Can you work these out from the model? Positions are in its coordinate system, mm. Coordinates: 2 decimals unless noted, no trailing zeros. Order: outer loops, then holes, each group sorted by start corner. A loop starts at its lowest first (then second) coordinate and runs counter-clockwise, first axis right, second up. Notation, with made-up numbers: (-16, 64) - (22, 64) arc R29 cw to (22, 94) - close; hole circle Ø9 at (-2.5, 34.25). An arc over 180 degrees is marked (long way). Use a Markdown table: item, result. Add a question column.
(1) I want a section at D-D (x = 29). List the corners of the cut face in (y, z) for me (3 decimals).
(2) If I drill on L1, parallel to Z at x = 19.05, y = 1; L2, parallel to X at y = 1.4, z = 12.7; L3, parallel to X at y = 0.75, z = 89, over which ranges is the centre line in solid material (lowest first)? Write a range as [from, to].
(3) I want a section at B-B (y = 1.7). List the corners of the cut face in (x, z) for me.
(4) I want a section at A-A (x = 19.05). List the corners of the cut face in (y, z) for me (3 decimals).
(5) I want a section at C-C (z = 20). List the corners of the cut face in (x, y) for me (3 decimals).
Autodesk Fusion 360 part; units mm, degrees
sketch "Sketch1" plane through (0, 0, 0) normal (0, 1, 0) x (1, 0, 0)
  arc A0 (38.1, -12.7) -> (0, -12.7) centre (19.05, -12.7) ccw
  line L0 (0, -12.7) -> (0, -88.9)
  line L1 (38.1, -12.7) -> (38.1, -88.9)
  arc A1 (0, -88.9) -> (38.1, -88.9) centre (19.05, -88.9) ccw
  dimension "d9" = 76.2
  dimension "d11" = 38.1
extrude "Extrude1" add sketch "Sketch1" along normal blind 3.175
hole "Hole1" at (19.05, 0, 88.9) direction (0, 1, 0) diameter 23.8125 end through all
hole "Hole2" at (19.05, 0, 12.7) direction (0, 1, 0) diameter 25.4 end through all
equation "stress = 9000 psi"
equation "d_A = 0.9375 in"
equation "d_1 = 1 in"
equation "d9 = Linear Dimension-2"
equation "d11 = Linear Dimension-3"
equation "d15 = d_A"
equation "d17 = d_1"
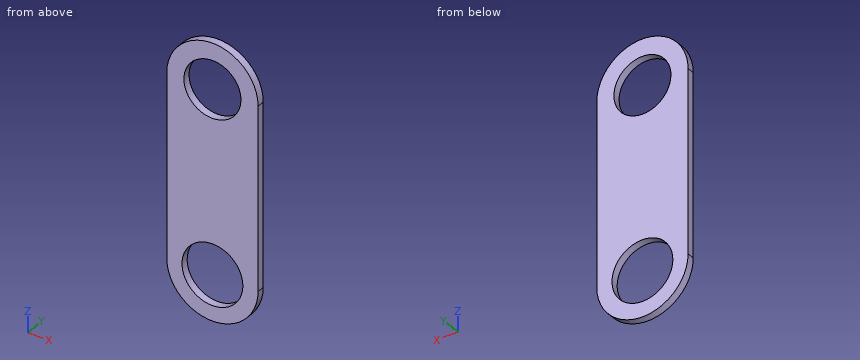
Answers follow:
| question | item | result |
|---|---|---|
| 1 | outline | (0, -3.545) - (3.175, -3.545) - (3.175, 4.808) - (0, 4.808) - close; (0, 20.592) - (3.175, 20.592) - (3.175, 82.361) - (0, 82.361) - close; (0, 95.439) - (3.175, 95.439) - (3.175, 105.145) - (0, 105.145) - close |
| 2 | L1 | z = [-6.35, 0], [25.4, 76.99], [100.81, 107.95] |
| 2 | L2 | x = [0, 6.35], [31.75, 38.1] |
| 2 | L3 | x = [0, 7.14], [30.96, 38.1] |
| 3 | outline | (0, 12.7) arc R19.05 ccw to (38.1, 12.7) - (38.1, 88.9) arc R19.05 ccw to (0, 88.9) - close; hole circle Ø25.4 at (19.05, 12.7); hole circle Ø23.81 at (19.05, 88.9) |
| 4 | outline | (0, -6.35) - (3.175, -6.35) - (3.175, 0) - (0, 0) - close; (0, 25.4) - (3.175, 25.4) - (3.175, 76.994) - (0, 76.994) - close; (0, 100.806) - (3.175, 100.806) - (3.175, 107.95) - (0, 107.95) - close |
| 5 | outline | (0, 0) - (8.658, 0) - (8.658, 3.175) - (0, 3.175) - close; (29.442, 0) - (38.1, 0) - (38.1, 3.175) - (29.442, 3.175) - close |
